Verification items for the finished model (mm, model axes). Round coordinates to 2 decimals unless told otherwise and drop trailing zeros. Write each loop counter-clockwise with the first axis right and the second up, starting at its lowest first coordinate (ties: lowest second). Pieces come first, ordered by that corner, then holes. Notation, with made-up numbers: M 71.5,4.5 L 126.5,4.5 A28 cw 126.5,38.5 Z; hole C 21.5,-6 d11. An arc over 180 degrees is marked long. Answer in a Markdown table with one row per item. Add a question column.
1. Sectioned sample at B-B on z = 1.35. Count the separate pieces of the cut face and the enclosed holes in it, plus the area to 3 significant figures.
2. Go/stop test with a flat-tipped pin: pin 1 Ø3 at (x, y) = (45, 0) entering from +Z. Record where the tip stops, or that it passes through.
3. Material ranges on probe 1 along Y at (x, z) = (60, 0.9); probe 2 along Y at (x, z) = (30, 3.65); probe 3 along Z at (x, y) = (-46, 1), recorded low to high.
4. Sectioned sample at A-A on x = -60. Record the cut outline in (y, z), plus the area to 3 significant figures.
```python
from build123d import *

# Parameters (mm, degrees)
SKETCH_1_W                = 140
SKETCH_1_H                = 5
EXTRUDE_1_DEPTH           = 4.8
HOLE_WIZARD_1_D           = 2.4
HOLE_WIZARD_1_DEPTH       = 5.2
HOLE_WIZARD_1_CBORE_D     = 4.3
HOLE_WIZARD_1_CBORE_DEPTH = 2.3
HOLE_WIZARD_1_TIP         = 0.721032743


with BuildPart() as part:
    # 草图1 → 凸台-拉伸1 (new body)
    with BuildSketch(Plane.XY):
        Rectangle(SKETCH_1_W, SKETCH_1_H)
    extrude(amount=EXTRUDE_1_DEPTH)

    # 打孔尺寸(%根据)内六角圆柱头螺钉的类型1
    with Locations(Plane.XY.offset(4.8)):
        with Locations((-60, 0), (-45, 0), (-30, 0), (-15, 0), (0, 0), (15, 0), (30, 0), (45, 0), (60, 0)):
            CounterBoreHole(HOLE_WIZARD_1_D / 2, HOLE_WIZARD_1_CBORE_D / 2, HOLE_WIZARD_1_CBORE_DEPTH, depth=HOLE_WIZARD_1_DEPTH)
            with Locations((0, 0, -(HOLE_WIZARD_1_DEPTH + HOLE_WIZARD_1_TIP / 2))):  # 118° drill point
                Cone(0, HOLE_WIZARD_1_D / 2, HOLE_WIZARD_1_TIP, mode=Mode.SUBTRACT)


solid = part.part
```
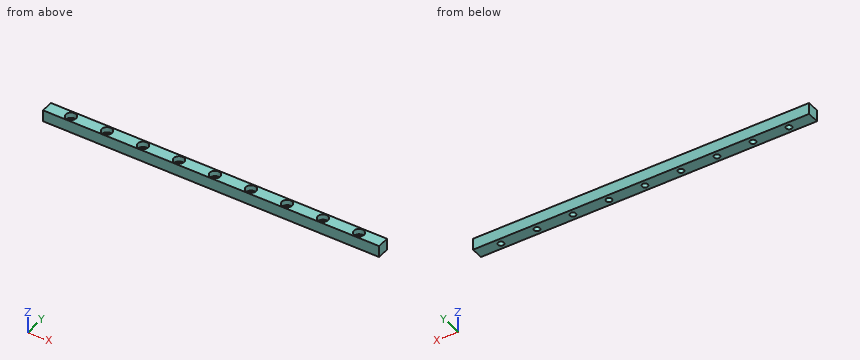
Geometry check:
| question | item | result |
|---|---|---|
| 1 | separate pieces | 1 |
| 1 | enclosed holes | 9 |
| 1 | area | 659 mm2 |
| 2 | pin 1 | stops at z = 2.5 |
| 3 | probe 1 | y = -2.5 to -1.2, 1.2 to 2.5 |
| 3 | probe 2 | y = -2.5 to -2.15, 2.15 to 2.5 |
| 3 | probe 3 | z = 0 to 2.5 |
| 4 | outline | M -2.5,0 L -1.2,0 L -1.2,2.5 L -2.15,2.5 L -2.15,4.8 L -2.5,4.8 Z; M 1.2,0 L 2.5,0 L 2.5,4.8 L 2.15,4.8 L 2.15,2.5 L 1.2,2.5 Z |
| 4 | area | 8.11 mm2 |
